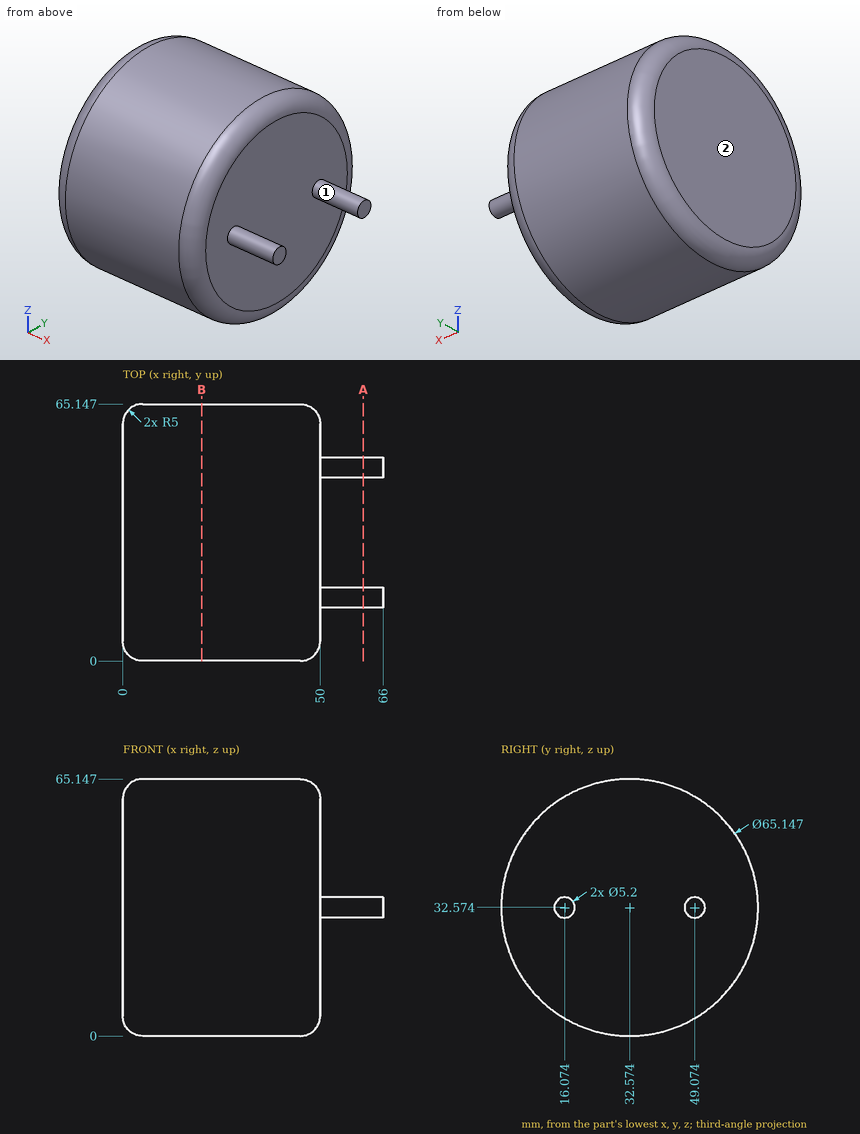
Input: dimensioned drawing with shaded views. Units: mm. Origin: part minimum x, y, z. A direction names the side the tool comes from. Coordinates: 2 decimals unless noted, no trailing zeros. Order: outer loops, then holes, each group sorted by start corner. A loop starts at its lowest first (then second) coordinate and runs counter-clockwise, first axis right, second up.
1. Ray query, line 1 along X through (y, z) = (45.5, 38); line 2 along Z through (x, y) = (46.5, 38); line 3 along Z through (x, y) = (21, 27). Return the intervals inside material, ascending.
Checked values:
line 1: x = 0 to 50
line 2: z = 0.69 to 64.46
line 3: z = 0.48 to 64.67
2. Access query for the marked faces 1 and 2. Directions: +Z, -Z, +X, -X, +Y, -Y. A direction counts if a zero-diameter tool reaches every point of the face in a straight line with its end or side. Return the directions, or none.
Checked values:
face 1: +X
face 2: +Z, -Z, -X, +Y, -Y
3. Cut plane A-A, the plane x = 61. Return loops of the section in (y, z).
Checked values:
outline: circle Ø5.2 at (16.07, 32.57); circle Ø5.2 at (49.07, 32.57)
4. Cut plane B-B, the plane x = 20. Return loops of the section in (y, z).
Checked values:
outline: circle Ø65.15 at (32.57, 32.57)
5. Contact query for flat-ended pins moving along their axis: P1, Ø8, axis at x = 43, y = 51, coming from the +Z side; P2, Ø4, axis at y = 35, z = 56, coming from the +X side; P3, Ø4, axis at y = 41.5, z = 35.5, coming from the -X side; P4, Ø12, axis at x = 38.5, y = 42.5, coming from the +Z side. Output: stop coordinate, or through.
Checked values:
P1: stops at z = 61.78
P2: stops at x = 50
P3: stops at x = 0
P4: stops at z = 64.91
